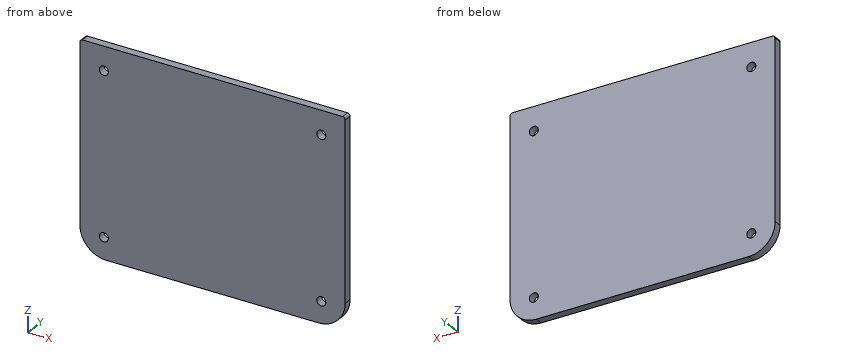
```python
from build123d import *

# Parameters (mm, degrees)
SKETCH1_W           = 100
SKETCH1_H           = 100
BOSS_EXTRUDE1_DEPTH = 3
SKETCH2_R           = 1.7
CUT_EXTRUDE1_DEPTH  = 3
SKETCH6_W           = 100
SKETCH6_H           = 21.808924231
CUT_EXTRUDE2_DEPTH  = 3
FILLET2_R           = 10
FILLET3_R           = 1


with BuildPart() as part:
    # Sketch1 → Boss-Extrude1 (new body)
    with BuildSketch(Plane(origin=(0, 33, 0), x_dir=(1, 0, 0), z_dir=(0, 1, 0))):
        Rectangle(SKETCH1_W, SKETCH1_H)
    extrude(amount=BOSS_EXTRUDE1_DEPTH)

    # Sketch2 → Cut-Extrude1 (cut)
    with BuildSketch(Plane(origin=(0, 36, 0), x_dir=(1, 0, 0), z_dir=(0, 1, 0))):
        with Locations(Location((-41, 20, 0), (0, 0, 270))):
            Circle(SKETCH2_R)
        with Locations(Location((41, 20, 0), (0, 0, 270))):
            Circle(SKETCH2_R)
        with Locations(Location((41, -41, 0), (0, 0, 270))):
            Circle(SKETCH2_R)
        with Locations(Location((-41, -41, 0), (0, 0, 270))):
            Circle(SKETCH2_R)
    extrude(amount=-CUT_EXTRUDE1_DEPTH, mode=Mode.SUBTRACT)

    # Sketch6 → Cut-Extrude2 (cut)
    with BuildSketch(Plane(origin=(0, 36, 0), x_dir=(1, 0, 0), z_dir=(0, 1, 0))):
        with Locations((0, 39.095537885)):
            Rectangle(SKETCH6_W, SKETCH6_H)
    extrude(amount=-CUT_EXTRUDE2_DEPTH, mode=Mode.SUBTRACT)

    # Fillet2
    fillet2_edges = [part.edges().sort_by_distance(p)[0] for p in [
        (-50, 34.5, -28.191075769),
        (50, 34.5, -28.191075769),
    ]]
    fillet(fillet2_edges, radius=FILLET2_R)

    # Fillet3
    fillet3_edges = [part.edges().sort_by_distance(p)[0] for p in [
        (50, 34.5, 50),
        (-50, 34.5, 50),
    ]]
    fillet(fillet3_edges, radius=FILLET3_R)


solid = part.part
```
CAD build for the part. Positions are in the model's coordinates, mm. Coordinates: 2 decimals unless noted, no trailing zeros. Write each loop counter-clockwise with the first axis right and the second up, starting at its lowest first coordinate (ties: lowest second). Pieces come first, ordered by that corner, then holes.
(1) Cut at A-A, the plane z = 41. List the corners of the cut face in (x, y), and give its area (3 significant figures).
(2) Flat gauge pin, fed straight in: pin 1 (2 mm diameter, centred on x = -41, z = 41, fed in from -Y). Where does the tip first touch, or does it go through?
(3) Cut at B-B, the plane z = -20. List the corners of the cut face in (x, y).
(4) Drill centre lines: probe 1 along X at (y, z) = (34.9, 41); probe 2 along X at (y, z) = (34.8, -21.5). Where is each one in solid material? Low to high.
Geometry says:
1. outline: (-50, 33) - (-42.7, 33) - (-42.7, 36) - (-50, 36) - close; (-39.3, 33) - (39.3, 33) - (39.3, 36) - (-39.3, 36) - close; (42.7, 33) - (50, 33) - (50, 36) - (42.7, 36) - close
1. area: 280 mm2
2. pin 1: passes through
3. outline: (-49.84, 33) - (-42.7, 33) - (-42.7, 36) - (-49.84, 36) - close; (-39.3, 33) - (39.3, 33) - (39.3, 36) - (-39.3, 36) - close; (42.7, 33) - (49.84, 33) - (49.84, 36) - (42.7, 36) - close
4. probe 1: x = -50 to -42.7, -39.3 to 39.3, 42.7 to 50
4. probe 2: x = -49.44 to -41.8, -40.2 to 40.2, 41.8 to 49.44
